Design review of the part shown in the three views and the two pictorial views. Dimensions are in mm from the part's minimum x, y and z. A direction names the side the tool comes from. Give positions to 0.01 mm unless a question says otherwise; leave off trailing zeros. Order: outer loops, then holes, each group sorted by start corner. A loop starts at its lowest first (then second) coordinate and runs counter-clockwise, first axis right, second up. Notation, with made-up numbers: (-8, 10.5) -> (25, 10.5) arc R29 ccw to (25, 44.5) -> close; hole circle Ø7 at (50, 80.5). An arc over 180 degrees is marked (long way). Answer in a Markdown table with one row per item. Add a question column.
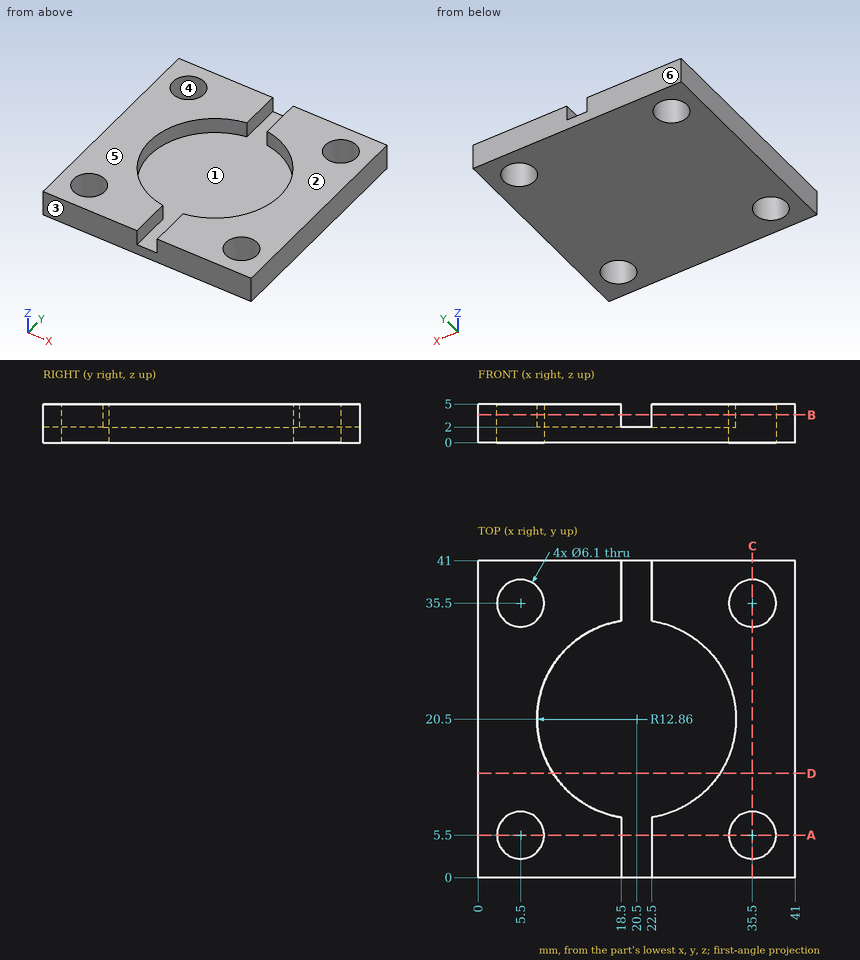
1) Add section C-C, the plane x = 35.5. Write out the cut boundary in (y, z), and give its area (3 significant figures).
2) Clearance check with a flat-ended pin moving along its axis: P1, Ø5.5, axis at x = 5.5, y = 35.5, coming from the +Z side. State where the tip first meets the part, or that it passes through.
3) Add section B-B, the plane z = 3.6. Write out the cut boundary in (x, y).
4) Add section D-D, the plane y = 13.5. Write out the cut boundary in (x, z), and give its area (3 significant figures).
5) Mouldability with a two-part tool opening along Y and no side actions: class the marked faces 3, 4, 5 and 6 as +Y half, -Y half, draft (parallel to the pull), parting line (faces both ways), or undercut.
6) For L1, parallel to Y at x = 35.5, z = 1.25; L2, parallel to Y at x = 6.5, z = 3.45; L3, parallel to Z at x = 16, y = 26, list the stretches that pass through material, from the lowest coordinate up.
7) Machinability: for the marked faces 1 and 2, which of the approach directions +Z, -Z, +X, -X, +Y, -Y give a long, thin tool a straight path to every point of the face, cutting with its end or side? Answer none if there is none.
8) Add section A-A, the plane y = 5.5. Write out the cut boundary in (x, z).
Verdict:
| question | item | result |
|---|---|---|
| 1 | outline | (0, 0) -> (2.45, 0) -> (2.45, 5) -> (0, 5) -> close; (8.55, 0) -> (32.45, 0) -> (32.45, 5) -> (8.55, 5) -> close; (38.55, 0) -> (41, 0) -> (41, 5) -> (38.55, 5) -> close |
| 1 | area | 144 mm2 |
| 2 | P1 | passes through |
| 3 | outline | (0, 0) -> (18.5, 0) -> (18.5, 7.8) arc R12.86 cw to (18.5, 33.2) -> (18.5, 41) -> (0, 41) -> close; (22.5, 0) -> (41, 0) -> (41, 41) -> (22.5, 41) -> (22.5, 33.2) arc R12.86 cw to (22.5, 7.8) -> close; hole circle Ø6.1 at (5.5, 5.5); hole circle Ø6.1 at (5.5, 35.5); hole circle Ø6.1 at (35.5, 5.5); hole circle Ø6.1 at (35.5, 35.5) |
| 4 | outline | (0, 0) -> (41, 0) -> (41, 5) -> (31.29, 5) -> (31.29, 2) -> (9.71, 2) -> (9.71, 5) -> (0, 5) -> close |
| 4 | area | 140 mm2 |
| 5 | face 3 | -Y half |
| 5 | face 4 | undercut |
| 5 | face 5 | draft |
| 5 | face 6 | +Y half |
| 6 | L1 | y = 0 to 2.45, 8.55 to 32.45, 38.55 to 41 |
| 6 | L2 | y = 0 to 2.62, 8.38 to 32.62, 38.38 to 41 |
| 6 | L3 | z = 0 to 2 |
| 7 | face 1 | +Z |
| 7 | face 2 | +Z, +X, -X, +Y, -Y |
| 8 | outline | (0, 0) -> (2.45, 0) -> (2.45, 5) -> (0, 5) -> close; (8.55, 0) -> (32.45, 0) -> (32.45, 5) -> (22.5, 5) -> (22.5, 2) -> (18.5, 2) -> (18.5, 5) -> (8.55, 5) -> close; (38.55, 0) -> (41, 0) -> (41, 5) -> (38.55, 5) -> close |
